Check sheet for the modelled part. Datum: model origin and axes. Units: mm. Face numbers are marked on the shaded views. Coordinates: 2 decimals unless noted, no trailing zeros. Write each loop counter-clockwise with the first axis right and the second up, starting at its lowest first coordinate (ties: lowest second). Pieces come first, ordered by that corner, then holes. Notation, with made-up numbers: (81.25, 30.25) -> (138.25, 30.25) arc R19 cw to (138.25, 66.25) -> close; hole circle Ø7 at (64.5, -11.75). An arc over 180 degrees is marked (long way). Put each result on its own line as item: value.
```python
from build123d import *

# Parameters (mm, degrees)
F0_W      = 95.9
F0_H      = 183
F1_DEPTH  = 9.8
F2_T      = -1.2
F3_SIZE   = 0.5
F4_SIZE   = 0.5
F5_SIZE   = 0.5
F6_SIZE   = 0.5
F7_SIZE   = 0.5
F8_SIZE   = 0.5
F9_SIZE   = 0.5
F11_DEPTH = 1.2
F13_DEPTH = 1.2
F15_ANGLE = 180
F16_ANGLE = 180
F18_ANGLE = 180
F19_ANGLE = 180
F20_DEPTH = 1


with BuildPart() as f1:
    # F0 (on Top) → F1 (new body)
    with BuildSketch(Plane.XY):
        with Locations((13.8901774406, 31.2419057786)):
            Rectangle(F0_W, F0_H)
    extrude(amount=F1_DEPTH)

    # F2
    f2_openings = [f1.faces().sort_by_distance(p)[0] for p in [
        (13.890177, 31.241906, 9.8),
    ]]
    offset(amount=F2_T, openings=f2_openings)

    # F3
    f3_edges = [f1.edges().sort_by_distance(p)[0] for p in [
        (61.840177, -60.258094, 4.9),
    ]]
    chamfer(f3_edges, length=F3_SIZE)

    # F4
    f4_edges = [f1.edges().sort_by_distance(p)[0] for p in [
        (-34.059823, -60.258094, 4.9),
    ]]
    chamfer(f4_edges, length=F4_SIZE)

    # F5
    f5_edges = [f1.edges().sort_by_distance(p)[0] for p in [
        (-34.059823, 122.741906, 4.9),
    ]]
    chamfer(f5_edges, length=F5_SIZE)

    # F6
    f6_edges = [f1.edges().sort_by_distance(p)[0] for p in [
        (61.840177, 122.741906, 4.9),
    ]]
    chamfer(f6_edges, length=F6_SIZE)

    # F7
    f7_edges = [f1.edges().sort_by_distance(p)[0] for p in [
        (60.640177, 121.541906, 5.5),
    ]]
    chamfer(f7_edges, length=F7_SIZE)

    # F8
    f8_edges = [f1.edges().sort_by_distance(p)[0] for p in [
        (-32.859823, 121.541906, 5.5),
    ]]
    chamfer(f8_edges, length=F8_SIZE)

    # F9
    f9_edges = [f1.edges().sort_by_distance(p)[0] for p in [
        (60.640177, -59.058094, 5.5),
        (-32.859823, -59.058094, 5.5),
    ]]
    chamfer(f9_edges, length=F9_SIZE)

    # F10 (on face) → F11 (join, through all)
    with BuildSketch(Plane.YZ.offset(61.8401774406)):
        Polygon((-51.0580942214, 18.5), (-59.7580942214, 9.8), (122.2419057786, 9.8), (113.5419057786, 18.5), align=None)
    extrude(amount=-F11_DEPTH)

    # F12 (on face) → F13 (join, through all)
    with BuildSketch(Plane(origin=(-34.0598225594, 0, 0), x_dir=(0, -1, 0), z_dir=(-1, 0, 0))):
        Polygon((51.0580942214, 18.5), (-113.5419057786, 18.5), (-122.2419057786, 9.8), (59.7580942214, 9.8), align=None)
    extrude(amount=-F13_DEPTH)

    # F14 (on face) → F15 (revolve)
    with BuildSketch(Plane.YZ.offset(-32.8598225594)):
        with BuildLine():
            Line((-15.5580942214, 13.3), (-13.0580942214, 13.3))
            ThreePointArc((-13.0580942214, 13.3), (-15.5580942214, 15.8), (-18.0580942214, 13.3))
            Line((-18.0580942214, 13.3), (-15.5580942214, 13.3))
        make_face()
    revolve(axis=Axis((-32.8598225594, -14.3080942214, 13.3), (0, 1, 0)), revolution_arc=F15_ANGLE)

    # F14 (on face) → F16 (revolve)
    with BuildSketch(Plane.YZ.offset(-32.8598225594)):
        with BuildLine():
            Line((78.0419057786, 13.3), (80.5419057786, 13.3))
            ThreePointArc((80.5419057786, 13.3), (78.0419057786, 15.8), (75.5419057786, 13.3))
            Line((75.5419057786, 13.3), (78.0419057786, 13.3))
        make_face()
    revolve(axis=Axis((-32.8598225594, 79.2919057786, 13.3), (0, 1, 0)), revolution_arc=F16_ANGLE)

    # F17 (on face) → F18 (revolve)
    with BuildSketch(Plane(origin=(60.6401774406, 0, 0), x_dir=(0, -1, 0), z_dir=(-1, 0, 0))):
        with BuildLine():
            Line((-78.0419057786, 13.3), (-75.5419057786, 13.3))
            ThreePointArc((-75.5419057786, 13.3), (-78.0419057786, 15.8), (-80.5419057786, 13.3))
            Line((-80.5419057786, 13.3), (-78.0419057786, 13.3))
        make_face()
    revolve(axis=Axis((60.6401774406, 76.7919057786, 13.3), (0, -1, 0)), revolution_arc=F18_ANGLE)

    # F17 (on face) → F19 (revolve)
    with BuildSketch(Plane(origin=(60.6401774406, 0, 0), x_dir=(0, -1, 0), z_dir=(-1, 0, 0))):
        with BuildLine():
            Line((15.5580942214, 13.3), (18.0580942214, 13.3))
            ThreePointArc((18.0580942214, 13.3), (15.5580942214, 15.8), (13.0580942214, 13.3))
            Line((13.0580942214, 13.3), (15.5580942214, 13.3))
        make_face()
    revolve(axis=Axis((60.6401774406, -16.8080942214, 13.3), (0, -1, 0)), revolution_arc=F19_ANGLE)

    # F20 (add): a face of the model
    f20_faces = [f1.faces().sort_by_distance(p)[0] for p in [
        (13.8901774406, 31.2419057786, 0),
    ]]
    extrude(f20_faces, amount=F20_DEPTH)


solid = f1.part
```
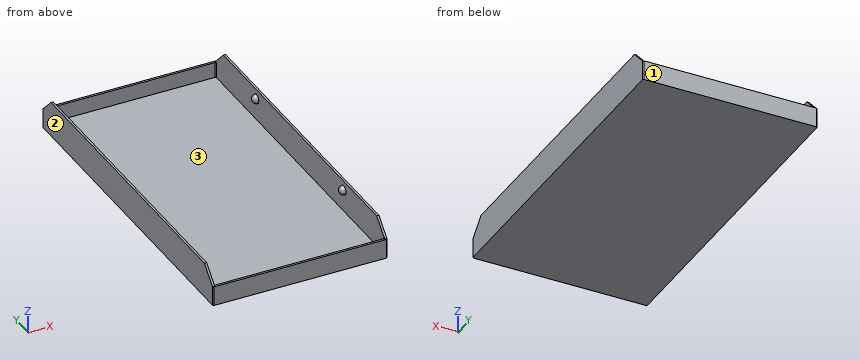
Q1. Mould release check, pull along Y, two halves, no side actions. Record for the marked faces 1, 2 and 3: released by +Y, released by -Y, zero draft, split by the parting line, or undercut.
Recorded:
face 1: released by +Y
face 2: zero draft
face 3: undercut
Q2. Cross-section at C-C (y = -46.5). Record the cut outline in (x, z), plus the area to 4 significant figures.
Recorded:
outline: (-34.06, -1) -> (61.84, -1) -> (61.84, 18.5) -> (60.64, 18.5) -> (60.64, 1.2) -> (-32.86, 1.2) -> (-32.86, 18.5) -> (-34.06, 18.5) -> close
area: 252.5 mm2
Q3. Material ranges on line 1 along Y through (x, z) = (33, 2.25); line 2 along X through (y, z) = (19, 2.25); line 3 along Z through (x, y) = (-12.5, -50), recorded low to high.
Recorded:
line 1: y = -60.26 to -59.06, 121.54 to 122.74
line 2: x = -34.06 to -32.86, 60.64 to 61.84
line 3: z = -1 to 1.2
Q4. Depth check by flat-ended pin: P1, Ø1.4, axis at x = 32, y = -59.5, coming from the +Z side; P2, Ø6, axis at x = -11.5, y = -25, coming from the +Z side; P3, Ø6, axis at x = 22, z = 15.5, coming from the +Y side. Enter the tip coordinate at first touch or a pass-through.
Recorded:
P1: stops at z = 9.8
P2: stops at z = 1.2
P3: passes through
Q5. Cross-section at A-A (z = 4). Record the cut outline in (x, y).
Recorded:
outline: (-34.06, -59.76) -> (-33.56, -60.26) -> (61.34, -60.26) -> (61.84, -59.76) -> (61.84, 122.24) -> (61.34, 122.74) -> (-33.56, 122.74) -> (-34.06, 122.24) -> close; hole (-32.86, -58.56) -> (-32.36, -59.06) -> (60.14, -59.06) -> (60.64, -58.56) -> (60.64, 121.04) -> (60.14, 121.54) -> (-32.36, 121.54) -> (-32.86, 121.04) -> close
Q6. Cross-section at B-B (x = 30). Record the cut outline in (y, z), plus the area to 3 significant figures.
Recorded:
outline: (-60.26, -1) -> (122.74, -1) -> (122.74, 9.8) -> (121.54, 9.8) -> (121.54, 1.2) -> (-59.06, 1.2) -> (-59.06, 9.8) -> (-60.26, 9.8) -> close
area: 423 mm2
